Autodesk Fusion 360 part; units mm, degrees
sketch "Sketch1" plane through (0, 0, 0) normal (0, 1, 0) x (1, 0, 0)
  line L0 (0, 0) -> (0, -19)
  line L1 (0, -19) -> (20, -19)
  line L2 (20, -19) -> (20, 0)
  line L3 (20, 0) -> (0, 0)
  line L4 (0, 0) -> (-3, 0)
  line L5 (-3, 0) -> (-3, 1)
  line L6 (-3, 1) -> (23, 1)
  line L7 (20, 0) -> (23, 0)
  line L8 (23, 0) -> (23, 1)
  dimension "d1" = 19
  dimension "d2" = 20
  dimension "d7" = 3
  dimension "d8" = 3
  dimension "d9" = 1
revolve "Revolve1" add sketch "Sketch1" angle 360 about axis through (20, 0, 0) along (-1, 0, 0) contours L3 L4 L5 L6 L7 L8
extrude "Extrude1" add sketch "Sketch1" along normal mid plane 2 contours L0 L1 L2 L3
equation "d8 = d7"
Input: part model. Units: mm. Frame: model coordinates. Coordinates: 2 decimals unless noted, no trailing zeros. Loops run counter-clockwise (first coordinate to the right, second up) from the corner with the lowest first, then second, coordinate; pieces in that order, holes last. Notation, with made-up numbers: (-2.75, -14) - (10.25, -14) arc R17 cw to (10.25, -5) - close; hole circle Ø6 at (-19.5, 18). An arc over 180 degrees is marked (long way). Answer in a Markdown table with one row per item. Add a question column.
Item 1: Section query B-B on z = 2.25. Return the cut outline in (x, y), then the cut area to 3 significant figures.
Item 2: Line query: line 1 along X through (y, z) = (-0.35, 4.5); line 2 along Z through (x, y) = (-0.75, 0.1); line 3 along Z through (x, y) = (2.75, 0.2). Output: solid intervals per line, ascending. Write a range as [from, to].
Item 3: Section query A-A on y = 0. Return the cut outline in (x, z), then the cut area to 3 significant figures.
Item 4: Contact query for a flat-ended pin moving along its axis: P1, Ø0.6, axis at y = 0, z = 10.5, coming from the -X side. Output: stop coordinate, or through.
Recorded:
| question | item | result |
|---|---|---|
| 1 | outline | (0, -1) - (20, -1) - (20, 1) - (0, 1) - close |
| 1 | area | 40.0 mm^2 |
| 2 | line 1 | [0, 20] |
| 2 | line 2 | [-0.99, 0.99] |
| 2 | line 3 | [-0.98, 19] |
| 3 | outline | (-3, -1) - (23, -1) - (23, 1) - (20, 1) - (20, 19) - (0, 19) - (0, 1) - (-3, 1) - close |
| 3 | area | 412 mm^2 |
| 4 | P1 | x = 0 |
